For this review, take the finished solid that the model builds, in its own axes (mm). Round coordinates to 2 decimals unless told otherwise and drop trailing zeros. Order: outer loops, then holes, each group sorted by start corner. A loop starts at its lowest first (then second) coordinate and runs counter-clockwise, first axis right, second up. Notation, with made-up numbers: (0.5, -10) - (14.5, -10) arc R14 ccw to (14.5, 2) - close; hole circle Ø11 at (49, -38). An arc over 180 degrees is marked (long way). One line per item, written item: value.
```python
from build123d import *

# Parameters (mm, degrees)
ESBO_O1_W                = 2.5
ESBO_O1_H                = 0.463123709
ESBO_O1_W_2              = 0.5
ESBO_O2_R                = 0.4
RESSALTO_EXTRUS_O1_DEPTH = 7
ESBO_O3_R                = 0.4
RESSALTO_EXTRUS_O2_DEPTH = 1
ESBO_O4_R                = 0.4
RESSALTO_EXTRUS_O3_DEPTH = 2


with BuildPart() as part:
    # Esboço1 → Revolução1 (revolve)
    with BuildSketch(Plane.XY):
        with BuildLine():
            Line((0, 7.133898305), (0, 4.633898305))
            ThreePointArc((0, 4.633898305), (1.767766953, 5.366131352), (2.5, 7.133898305))
            Line((2.5, 7.133898305), (0, 7.133898305))
        make_face()
        with BuildLine():
            Line((0, 9.633898305), (0, 7.133898305))
            Line((0, 7.133898305), (2.5, 7.133898305))
            ThreePointArc((2.5, 7.133898305), (1.767766953, 8.901665258), (0, 9.633898305))
        make_face()
        with BuildLine():
            Line((0, 7.133898305), (0, 4.633898305))
            ThreePointArc((0, 4.633898305), (1.767766953, 5.366131352), (2.5, 7.133898305))
            Line((2.5, 7.133898305), (0, 7.133898305))
        make_face()
        with BuildLine():
            Line((0, 9.633898305), (0, 7.133898305))
            Line((0, 7.133898305), (2.5, 7.133898305))
            ThreePointArc((2.5, 7.133898305), (1.767766953, 8.901665258), (0, 9.633898305))
        make_face()
        with BuildLine():
            Line((0, 4.633898305), (0, 1.497022014))
            Line((0, 1.497022014), (2.5, 1.497022014))
            Line((2.5, 1.497022014), (2.5, 7.133898305))
            ThreePointArc((2.5, 7.133898305), (1.767766953, 5.366131352), (0, 4.633898305))
        make_face()
        with Locations((1.25, 1.26546016)):
            Rectangle(ESBO_O1_W, ESBO_O1_H)
        with Locations((2.75, 1.26546016)):
            Rectangle(ESBO_O1_W_2, ESBO_O1_H)
    revolve(axis=Axis((0, 1.033898305, 0), (0, 1, 0)))

    # Esboço2 → Ressalto-extrusão1 (add)
    with BuildSketch(Plane.XZ.offset(-1.033898305)):
        with Locations((-1.5, 0)):
            Circle(ESBO_O2_R)
        with Locations((-0.5, 0)):
            Circle(ESBO_O2_R)
        with Locations((0.5, 0)):
            Circle(ESBO_O2_R)
        with Locations((1.5, 0)):
            Circle(ESBO_O2_R)
    extrude(amount=RESSALTO_EXTRUS_O1_DEPTH)

    # Esboço3 → Ressalto-extrusão2 (add)
    with BuildSketch(Plane.XZ.offset(5.966101695)):
        with Locations((0.5, 0)):
            Circle(ESBO_O3_R)
        with Locations((-1.5, 0)):
            Circle(ESBO_O3_R)
    extrude(amount=RESSALTO_EXTRUS_O2_DEPTH)

    # Esboço4 → Ressalto-extrusão3 (add)
    with BuildSketch(Plane.XZ.offset(5.966101695)):
        with Locations((-0.5, 0)):
            Circle(ESBO_O4_R)
    extrude(amount=RESSALTO_EXTRUS_O3_DEPTH)


solid = part.part
```
Item 1: Take a section at A-A (z = 0). Write out the cut boundary in (x, y), plus the area to 3 significant figures.
Returned:
outline: (-3, 1.03) - (-1.9, 1.03) - (-1.9, -6.97) - (-1.1, -6.97) - (-1.1, 1.03) - (-0.9, 1.03) - (-0.9, -7.97) - (-0.1, -7.97) - (-0.1, 1.03) - (0.1, 1.03) - (0.1, -6.97) - (0.9, -6.97) - (0.9, 1.03) - (1.1, 1.03) - (1.1, -5.97) - (1.9, -5.97) - (1.9, 1.03) - (3, 1.03) - (3, 1.5) - (2.5, 1.5) - (2.5, 7.13) arc R2.5 ccw to (-2.5, 7.13) - (-2.5, 1.5) - (-3, 1.5) - close
area: 66.4 mm^2
Item 2: The part is to be moulded in two halves that separate along Z. For faces 1 (the flat face through (2, 1.497, -2)), 2 (the cylindrical face through (-3, 1.3, -0.1)), say which applies: +Z half, -Z half, draft (parallel to the pull), parting line (faces both ways), or undercut.
Returned:
face 1: draft
face 2: parting line
Item 3: Take a section at B-B (y = -1.25). Write out the cut boundary in (x, z), plus the area to 3 significant figures.
Returned:
outline: circle Ø0.8 at (-1.5, 0); circle Ø0.8 at (-0.5, 0); circle Ø0.8 at (0.5, 0); circle Ø0.8 at (1.5, 0)
area: 2.01 mm^2
Item 4: Take a section at D-D (x = -1.5). Write out the cut boundary in (y, z), plus the area to 3 significant figures.
Returned:
outline: (-6.97, -0.4) - (1.03, -0.4) - (1.03, -2.6) - (1.5, -2.6) - (1.5, -2) - (7.13, -2) arc R2 ccw to (7.13, 2) - (1.5, 2) - (1.5, 2.6) - (1.03, 2.6) - (1.03, 0.4) - (-6.97, 0.4) - close
area: 37.6 mm^2
Item 5: For P1, Ø1, axis at x = -1.5, y = -2.5, coming from the -Z side; P2, Ø1, axis at y = -3, z = -0.5, coming from the -X side; P3, Ø1.5, axis at x = -1, z = -2.5, coming from the -Y side, all flat-tipped, find the tip position at first contact; note any pin that passes through.
Returned:
P1: z = -0.4
P2: x = -1.9
P3: y = 1.03
Item 6: Take a section at C-C (x = 1.5). Write out the cut boundary in (y, z).
Returned:
outline: (-5.97, -0.4) - (1.03, -0.4) - (1.03, -2.6) - (1.5, -2.6) - (1.5, -2) - (7.13, -2) arc R2 ccw to (7.13, 2) - (1.5, 2) - (1.5, 2.6) - (1.03, 2.6) - (1.03, 0.4) - (-5.97, 0.4) - close
Item 7: Wall thickness on line 1 (Y direction, x = 2.7, z = 0.5); line 2 (X direction, y = -2, z = -0.15); line 3 (X direction, y = 2.25, z = -0.15): over which ranges is each line inside the solid? List them lowest first.
Returned:
line 1: 1.03 to 1.5
line 2: -1.87 to -1.13, -0.87 to -0.13, 0.13 to 0.87, 1.13 to 1.87
line 3: -2.5 to 2.5
